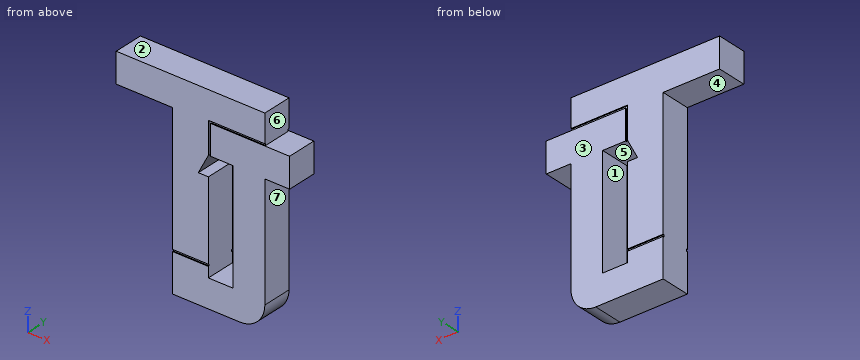
```python
from build123d import *

# Parameters (mm, degrees)
F0_W     = 9.144
F0_H     = 0.508
F1_DEPTH = 7.62
F2_DEPTH = 7.366
F3_DEPTH = 0.254
F4_W     = 9.144
F4_H     = 0.508
F5_DEPTH = 0.254


with BuildPart() as f1:
    # F0 (on Front) → F1 (new body)
    with BuildSketch(Plane.XZ):
        Polygon((-10.693384, 33.075266), (-48.793384, 33.075266), (-48.793384, 25.455266), (-34.315384, 25.455266), (-34.315384, -7.374234), (-25.171384, -7.374234), (-25.171384, 12.856693), (-27.764196, 12.856693), (-25.171384, 17.835266), (-25.171384, 25.137766), (-25.171384, 25.455266), (-25.171384, 25.963266), (-10.693384, 25.963266), align=None)
        with Locations((-29.743384, -7.628234)):
            Rectangle(F0_W, F0_H)
        with BuildLine():
            Line((-4.343384, 25.455266), (-10.693384, 25.455266))
            Line((-10.693384, 25.455266), (-24.663384, 25.455266))
            Line((-24.663384, 25.455266), (-24.663384, 17.835266))
            Line((-24.663384, 17.835266), (-18.821384, 17.835266))
            Line((-18.821384, 17.835266), (-18.821384, -10.542493))
            Line((-18.821384, -10.542493), (-25.171384, -10.542493))
            Line((-25.171384, -10.542493), (-25.171384, -7.882234))
            Line((-25.171384, -7.882234), (-34.315384, -7.882234))
            Line((-34.315384, -7.882234), (-34.315384, -17.724734))
            Line((-34.315384, -17.724734), (-17.043384, -17.724734))
            ThreePointArc((-17.043384, -17.724734), (-12.553256, -15.864862), (-10.693384, -11.374734))
            Line((-10.693384, -11.374734), (-10.693384, 17.835266))
            Line((-10.693384, 17.835266), (-4.343384, 17.835266))
            Line((-4.343384, 17.835266), (-4.343384, 25.455266))
        make_face()
    extrude(amount=-F1_DEPTH)

    # F0 (on Front) → F2 (join)
    with BuildSketch(Plane.XZ):
        Polygon((-10.693384, 25.455266), (-10.693384, 25.963266), (-25.171384, 25.963266), (-25.171384, 25.455266), (-24.663384, 25.455266), align=None)
        Polygon((-24.663384, 25.455266), (-25.171384, 25.455266), (-25.171384, 25.137766), (-25.171384, 17.835266), (-24.663384, 17.835266), align=None)
        with Locations((-29.743384, -7.628234)):
            Rectangle(F0_W, F0_H)
    extrude(amount=-F2_DEPTH)

    # F0 (on Front) → F3 (cut)
    with BuildSketch(Plane.XZ):
        Polygon((-24.663384, 25.455266), (-25.171384, 25.455266), (-25.171384, 25.137766), (-25.171384, 17.835266), (-24.663384, 17.835266), align=None)
        Polygon((-10.693384, 25.455266), (-10.693384, 25.963266), (-25.171384, 25.963266), (-25.171384, 25.455266), (-24.663384, 25.455266), align=None)
        with Locations((-29.743384, -7.628234)):
            Rectangle(F0_W, F0_H)
    extrude(amount=-F3_DEPTH, mode=Mode.SUBTRACT)

    # F4 (on face) → F5 (cut)
    with BuildSketch(Plane(origin=(0, 7.62, 0), x_dir=(-1, 0, 0), z_dir=(0, 1, 0))):
        with Locations((29.743384, -7.62705)):
            Rectangle(F4_W, F4_H)
    extrude(amount=-F5_DEPTH, mode=Mode.SUBTRACT)


solid = f1.part
```
CAD build for the part. Positions are in the model's coordinates, mm. Face numbers are marked on the shaded views. A direction names the side the tool comes from. Round coordinates to 2 decimals unless told otherwise and drop trailing zeros. Order: outer loops, then holes, each group sorted by start corner. A loop starts at its lowest first (then second) coordinate and runs counter-clockwise, first axis right, second up. Notation, with made-up numbers: (59, 70.5) - (88, 70.5) arc R21 cw to (88, 87.5) - close; hole circle Ø7 at (24, 40). An arc over 180 degrees is marked (long way). Answer as CSV lines item,"result". Start each with the question number.
1. Drill centre lines: L1, parallel to Z at x = -21, y = 4; L2, parallel to X at y = 2.5, z = -1; L3, parallel to Z at x = -41.5, y = 3.25. Where is each one in solid material? Low to high. Write a range as [from, to].
2. Pin check, flat tips, straight feed: pin 1 (4 mm diameter, centred on x = -41.5, y = 5, fed in from -Z); pin 2 (1.5 mm diameter, centred on y = 1.5, z = 16, fed in from +X). Stop position of each tip, or through.
3. Saw through at A-A, the plane z = -5. Write the cut outline in (x, y), and give its area (3 significant figures).
4. Pull direction Z, two halves, no side cores. Call the marked faces 1, 2 and 3: +Z half, -Z half, draft (parallel to the pull), parting line (faces both ways), or undercut.
5. Saw through at D-D, the plane x = -39.5. Write the cut outline in (y, z), and give its area (3 significant figures).
6. Saw through at B-B, the plane y = 1.75. Write the cut outline in (x, z).
7. Saw through at C-C, the plane z = 20.5. Write the cut outline in (x, y).
8. Tool access for the marked faces 4, 5, 6 and 7: list every direction of +Z, -Z, +X, -X, +Y, -Y with a clear straight run to the whole face (end or side of a thin tool).
Model answer:
1,L1,"z = [-17.72, -10.54], [17.84, 33.08]"
1,L2,"x = [-34.32, -25.17], [-18.82, -10.69]"
1,L3,"z = [25.46, 33.08]"
2,pin 1,"stops at z = 25.46"
2,pin 2,"stops at x = -10.69"
3,outline,"(-34.32, 0) - (-25.17, 0) - (-25.17, 7.62) - (-34.32, 7.62) - close; (-18.82, 0) - (-10.69, 0) - (-10.69, 7.62) - (-18.82, 7.62) - close"
3,area,"132 mm²"
4,face 1,"undercut"
4,face 2,"+Z half"
4,face 3,"draft"
5,outline,"(0, 25.46) - (7.62, 25.46) - (7.62, 33.08) - (0, 33.08) - close"
5,area,"58.1 mm²"
6,outline,"(-48.79, 25.46) - (-34.32, 25.46) - (-34.32, -17.72) - (-17.04, -17.72) arc R6.35 ccw to (-10.69, -11.37) - (-10.69, 17.84) - (-4.34, 17.84) - (-4.34, 25.46) - (-10.69, 25.46) - (-10.69, 33.08) - (-48.79, 33.08) - close; hole (-27.76, 12.86) - (-25.17, 12.86) - (-25.17, -10.54) - (-18.82, -10.54) - (-18.82, 17.84) - (-25.17, 17.84) - close"
7,outline,"(-34.32, 0) - (-25.17, 0) - (-25.17, 0.25) - (-24.66, 0.25) - (-24.66, 0) - (-4.34, 0) - (-4.34, 7.62) - (-24.66, 7.62) - (-24.66, 7.37) - (-25.17, 7.37) - (-25.17, 7.62) - (-34.32, 7.62) - close"
8,face 4,"-Z, -X, +Y, -Y"
8,face 5,"+Y, -Y"
8,face 6,"+Z, +X, +Y, -Y"
8,face 7,"-Z, +X, +Y, -Y"
